The model under review builds one solid part; all positions refer to its coordinate system, in mm. Round coordinates to 2 decimals unless told otherwise and drop trailing zeros. Write each loop counter-clockwise with the first axis right and the second up, starting at its lowest first coordinate (ties: lowest second). Pieces come first, ordered by that corner, then holes. Notation, with made-up numbers: M 26.25,11 L 36.25,11 A13 cw 36.25,36 Z; hole C -16,8.5 d4. An arc over 180 degrees is marked long. One line per item, written item: value. Start each with the question number.
1) Take a section at C-C, the plane x = 0. Write out the cut boundary in (y, z).
2) Take a section at D-D, the plane z = 0.7. Write out the cut boundary in (x, y), and give its area (3 significant figures).
3) For P1, Ø1.5, axis at x = 16.5, y = -6, coming from the +Z side; P2, Ø0.8, axis at x = 0, z = 0.5, coming from the +Y side; P3, Ø0.8, axis at x = -3, z = 1, coming from the -Y side, all flat-tipped, find the tip position at first contact; note any pin that passes through.
4) Take a section at A-A, the plane x = -16.5. Write out the cut boundary in (y, z), and give its area (3 significant figures).
5) Take a section at B-B, the plane y = 0. Write out the cut boundary in (x, z).
6) Wall thickness on probe 1 along Y at (x, z) = (-16, 0.3); probe 2 along Y at (x, z) = (-16.5, 0.55); probe 3 along X at (y, z) = (-5.5, 0.6): over which ranges is each line inside the solid? List them lowest first.
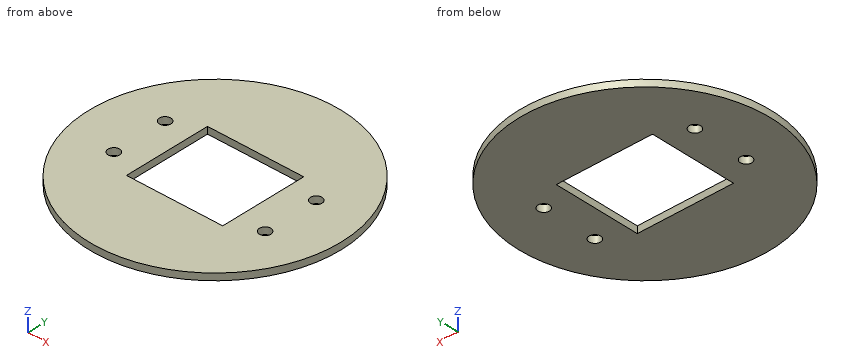
from build123d import *

# Parameters (mm, degrees)
SKETCH_2_R          = 27.5
SKETCH_2_W          = 21
SKETCH_2_H          = 19
EXTRUDE_2_DEPTH     = 1.5
SKETCH_3_R          = 1.25
CUT_EXTRUDE_1_DEPTH = 10


with BuildPart() as part:
    # 草图2 → 凸台-拉伸2 (new body)
    with BuildSketch(Plane.XY):
        Circle(SKETCH_2_R)
        Rectangle(SKETCH_2_W, SKETCH_2_H, mode=Mode.SUBTRACT)
    extrude(amount=EXTRUDE_2_DEPTH)

    # 草图3 → 切除-拉伸1 (cut)
    with BuildSketch(Plane.XY.offset(1.5)):
        with Locations((16.5, 6)):
            Circle(SKETCH_3_R)
        with Locations((-16.5, 6)):
            Circle(SKETCH_3_R)
        with Locations((16.5, -6)):
            Circle(SKETCH_3_R)
        with Locations((-16.5, -6)):
            Circle(SKETCH_3_R)
    extrude(amount=-CUT_EXTRUDE_1_DEPTH, mode=Mode.SUBTRACT)


solid = part.part
Checked values:
1. outline: M -27.5,0 L -9.5,0 L -9.5,1.5 L -27.5,1.5 Z; M 9.5,0 L 27.5,0 L 27.5,1.5 L 9.5,1.5 Z
2. outline: C 0,0 d55; hole C -16.5,-6 d2.5; hole C -16.5,6 d2.5; hole M -10.5,-9.5 L 10.5,-9.5 L 10.5,9.5 L -10.5,9.5 Z; hole C 16.5,-6 d2.5; hole C 16.5,6 d2.5
2. area: 1,960 mm2
3. P1: passes through
3. P2: stops at y = 27.5
3. P3: stops at y = -27.38
4. outline: M -22,0 L -7.25,0 L -7.25,1.5 L -22,1.5 Z; M -4.75,0 L 4.75,0 L 4.75,1.5 L -4.75,1.5 Z; M 7.25,0 L 22,0 L 22,1.5 L 7.25,1.5 Z
4. area: 58.5 mm2
5. outline: M -27.5,0 L -10.5,0 L -10.5,1.5 L -27.5,1.5 Z; M 10.5,0 L 27.5,0 L 27.5,1.5 L 10.5,1.5 Z
6. probe 1: y = -22.37 to -7.15, -4.85 to 4.85, 7.15 to 22.37
6. probe 2: y = -22 to -7.25, -4.75 to 4.75, 7.25 to 22
6. probe 3: x = -26.94 to -17.65, -15.35 to -10.5, 10.5 to 15.35, 17.65 to 26.94
